Source: three-view drawing plus pictorial views. Frame: mm from the lowest corner of the part. A direction names the side the tool comes from. Give positions to 0.01 mm unless a question says otherwise; leave off trailing zeros. Loops run counter-clockwise (first coordinate to the right, second up) from the corner with the lowest first, then second, coordinate; pieces in that order, holes last. Notation, with made-up numbers: (60, -18) - (105, -18) arc R21 cw to (105, 5) - close; hole circle Ø7 at (27, -30). An arc over 180 degrees is marked (long way). Put each result on its own line as item: value.
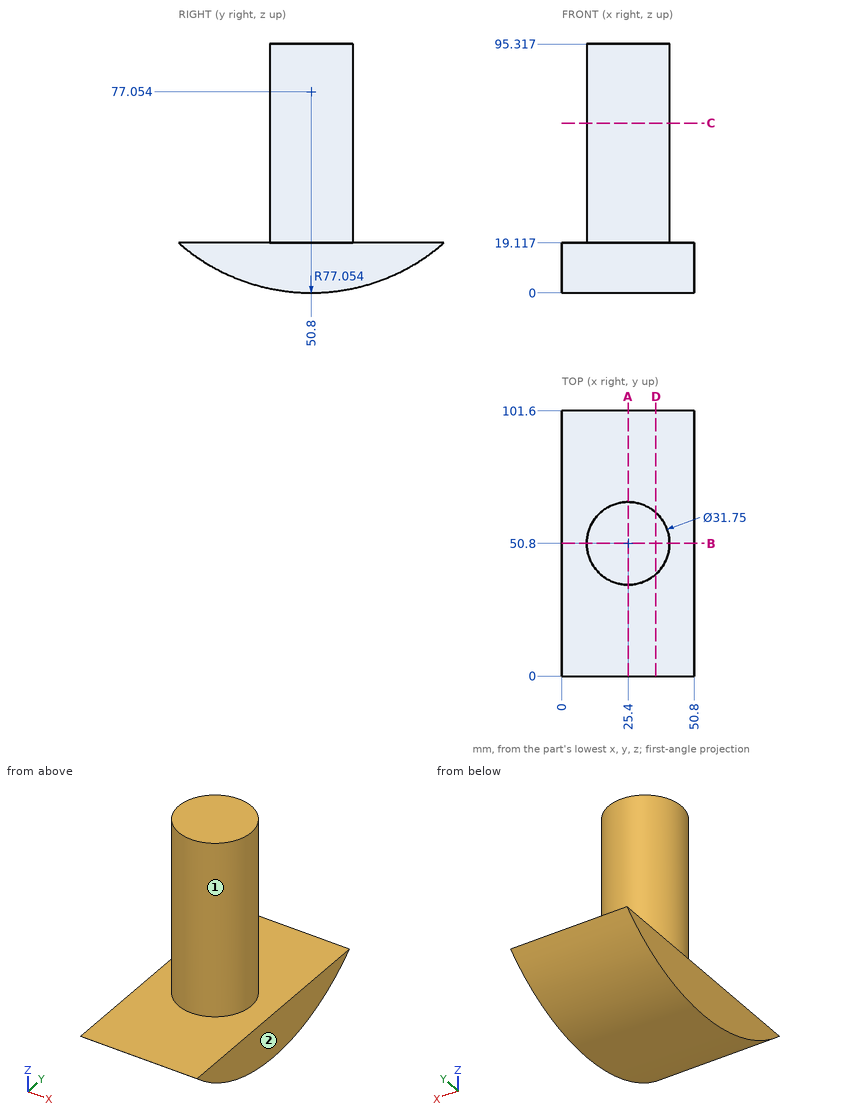
1) Section query A-A, the plane x = 25.4. Output: boundary loops of the cut face in (y, z) (1 decimal).
Check result:
outline: (0, 19.1) arc R77.1 ccw to (101.6, 19.1) - (66.7, 19.1) - (66.7, 95.3) - (34.9, 95.3) - (34.9, 19.1) - close
2) Section query C-C, the plane z = 65. Output: boundary loops of the cut face in (x, y) (3 decimals), plus the area to 3 significant figures.
Check result:
outline: circle Ø31.75 at (25.4, 50.8)
area: 792 mm²
3) Material intervals for line 1 along Y through (x, z) = (25, 51); line 2 along Z through (x, y) = (4.5, 87); line 3 along Z through (x, y) = (45, 51), sorted ascending. Write a range as [from, to].
Check result:
line 1: [34.93, 66.67]
line 2: [9.03, 19.12]
line 3: [0, 19.12]
4) Section query B-B, the plane y = 50.8. Output: boundary loops of the cut face in (x, z) (1 decimal), plus the area to 3 significant figures.
Check result:
outline: (0, 0) - (50.8, 0) - (50.8, 19.1) - (41.3, 19.1) - (41.3, 95.3) - (9.5, 95.3) - (9.5, 19.1) - (0, 19.1) - close
area: 3,390 mm²
5) Section query D-D, the plane x = 36. Output: boundary loops of the cut face in (y, z), plus the area to 3 significant figures.
Check result:
outline: (0, 19.12) arc R77.05 ccw to (101.6, 19.12) - (62.62, 19.12) - (62.62, 95.32) - (38.98, 95.32) - (38.98, 19.12) - close
area: 3,130 mm²
6) Access query for the marked faces 1 and 2. Directions: +Z, -Z, +X, -X, +Y, -Y. A direction counts if a zero-diameter tool reaches every point of the face in a straight line with its end or side. Return the directions, or none.
Check result:
face 1: +Z
face 2: +Z, -Z, +X, +Y, -Y
7) Pin query (flat end, axial travel): P1, Ø1.5, axis at x = 34.5, z = 72, coming from the -Y side; P2, Ø12, axis at x = 34, z = 47, coming from the -Y side; P3, Ø5, axis at x = 25, y = 44, coming from the -Z side. Return the tip coordinate at first contact, or that it passes through.
Check result:
P1: y = 37.3
P2: y = 35.14
P3: z = 0.12
